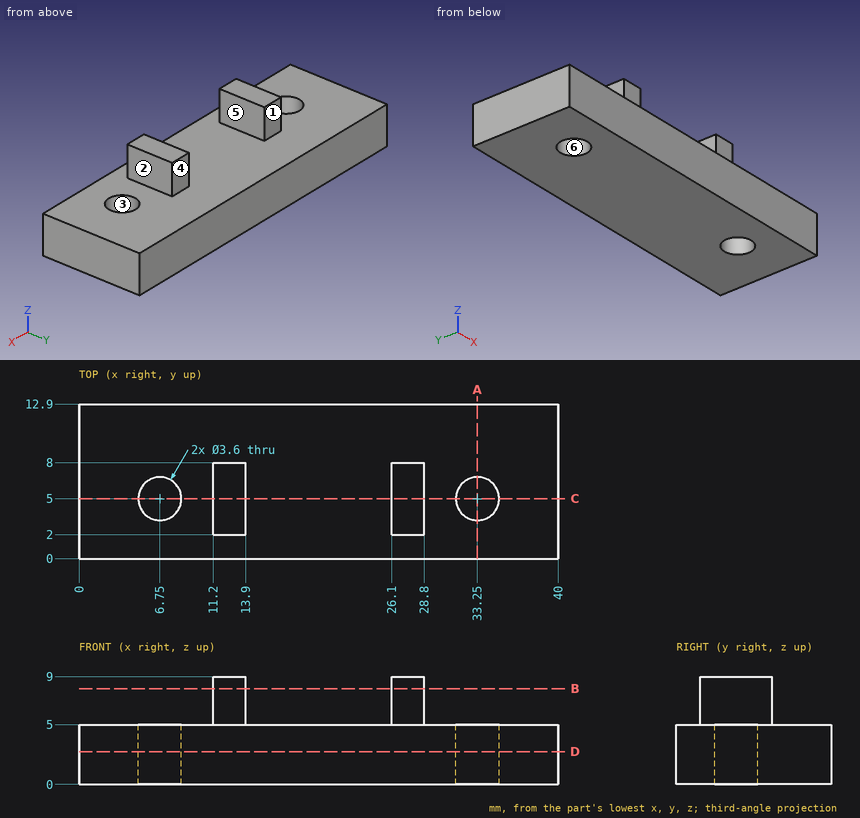
Can you work these out from the drawing? Everything is in mm from the part's minimum corner. A direction names the side the tool comes from. Round coordinates to 2 decimals unless told otherwise and drop trailing zeros. Write each loop counter-clockwise with the first axis right and the second up, starting at its lowest first coordinate (ties: lowest second). Pieces come first, ordered by that corner, then holes. Notation, with made-up numbers: M 84,66.5 L 130,66.5 A8 ccw 130,74.5 Z; hole C -16,40.5 d8. An arc over 180 degrees is marked long. Use a Markdown table: item, result.
Item 1: Which directions (+Z, -Z, +X, -X, +Y, -Y) give clear straight access to the entire face, cutting with the end or side of a thin tool? Please do the marked faces 4, 5 and 6.
Found:
| item | result |
|---|---|
| face 4 | +Z, +X, -X, +Y |
| face 5 | +Z, +Y, -Y |
| face 6 | +Z, -Z |
Item 2: We'd pull the mould along X, two halves only. Please class the marked faces 1, 2 and 3: released by +X, released by -X, zero draft, split by the parting line, or undercut.
Found:
| item | result |
|---|---|
| face 1 | zero draft |
| face 2 | released by +X |
| face 3 | undercut |
Item 3: I want a section at A-A (x = 33.25). List the corners of the cut face in (y, z) for me, and give its area (3 significant figures).
Found:
| item | result |
|---|---|
| outline | M 0,0 L 3.2,0 L 3.2,5 L 0,5 Z; M 6.8,0 L 12.9,0 L 12.9,5 L 6.8,5 Z |
| area | 46.5 mm2 |
Item 4: For pin 1 Ø2 at (y, z) = (3.5, 6.5) entering from -X; pin 2 Ø1.4 at (x, z) = (27.5, 7) entering from +Y; pin 3 Ø2 at (y, z) = (3.5, 8) entering from +X, each with a flat end and sliding along its axis, tell me the tip position at first contact or that it passes through.
Found:
| item | result |
|---|---|
| pin 1 | stops at x = 11.2 |
| pin 2 | stops at y = 8 |
| pin 3 | stops at x = 28.8 |
Item 5: If I drill on line 1 along X through (y, z) = (5, 3.1); line 2 along X through (y, z) = (7.25, 6.5); line 3 along Y through (x, z) = (6.75, 3.4), over which ranges is the centre line in solid material (lowest first)? Write a range as [from, to].
Found:
| item | result |
|---|---|
| line 1 | x = [0, 4.95], [8.55, 31.45], [35.05, 40] |
| line 2 | x = [11.2, 13.9], [26.1, 28.8] |
| line 3 | y = [0, 3.2], [6.8, 12.9] |
Item 6: I want a section at D-D (z = 2.75). List the corners of the cut face in (x, y) for me.
Found:
| item | result |
|---|---|
| outline | M 0,0 L 40,0 L 40,12.9 L 0,12.9 Z; hole C 6.75,5 d3.6; hole C 33.25,5 d3.6 |
Item 7: I want a section at C-C (y = 5). List the corners of the cut face in (x, z) for me.
Found:
| item | result |
|---|---|
| outline | M 0,0 L 4.95,0 L 4.95,5 L 0,5 Z; M 8.55,0 L 31.45,0 L 31.45,5 L 28.8,5 L 28.8,9 L 26.1,9 L 26.1,5 L 13.9,5 L 13.9,9 L 11.2,9 L 11.2,5 L 8.55,5 Z; M 35.05,0 L 40,0 L 40,5 L 35.05,5 Z |
Item 8: I want a section at B-B (z = 8). List the corners of the cut face in (x, y) for me, and give its area (3 significant figures).
Found:
| item | result |
|---|---|
| outline | M 11.2,2 L 13.9,2 L 13.9,8 L 11.2,8 Z; M 26.1,2 L 28.8,2 L 28.8,8 L 26.1,8 Z |
| area | 32.4 mm2 |
